Autodesk Inventor part; units mm, degrees
ref_plane "YZ Plane" through (0, 0, 0) normal (1, 0, 0) x (0, 1, 0)
ref_plane "XZ Plane" through (0, 0, 0) normal (0, 1, 0) x (-1, 0, 0)
ref_plane "XY Plane" through (0, 0, 0) normal (0, 0, 1) x (1, 0, 0)
sketch "Sketch1" plane through (0, 0, 0) normal (0, 0, 1) x (1, 0, 0)
  line L0 (-160.1126, 202.6875) -> (-23.9126, 202.6875)
  line L1 (-23.9126, 202.6875) -> (-23.9126, 142.6875)
  line L2 (-23.9126, 142.6875) -> (-163.9126, 142.6875)
  line L3 (-163.9126, 142.6875) -> (-163.9126, 198.8875)
  circle A0 centre (-160.1126, 198.8875) radius 1.5
  arc A1 (-160.1126, 202.6875) -> (-163.9126, 198.8875) centre (-160.1126, 198.8875) ccw
  line L4 (-163.9126, 172.6875) -> (-23.9126, 172.6875) construction
  line L5 (-93.9126, 142.6875) -> (-93.9126, 202.6875) construction
  circle A2 centre (-160.1126, 146.4875) radius 1.5
  circle A3 centre (-27.7126, 198.8875) radius 1.5
  circle A4 centre (-27.7126, 146.4875) radius 1.5
  arc A5 (-163.9126, 146.4875) -> (-160.1126, 142.6875) centre (-160.1126, 146.4875) ccw
  arc A6 (-23.9126, 198.8875) -> (-27.7126, 202.6875) centre (-27.7126, 198.8875) ccw
  arc A7 (-27.7126, 142.6875) -> (-23.9126, 146.4875) centre (-27.7126, 146.4875) ccw
  point P0 (0, 0)
  point P1 (-163.9126, 202.6875)
  dimension "d0" = 60
  dimension "d1" = 140
  dimension "d2" = 3
  dimension "d3" = 3.8
  dimension "d4" = 3.8
  dimension "d5" = 3.8
extrude "Extrusion1" add sketch "Sketch1" along normal blind 1.6 contours L0 A6 L1 A7 L2 A5 L3 A1
sketch "Sketch2" plane through (0, 0, 0) normal (0, 0, -1) x (-1, 0, 0)
  line L0 (139.9626, 193.3375) -> (107.8626, 193.3375)
  line L1 (107.8626, 193.3375) -> (107.8626, 152.0375) construction
  line L2 (107.8626, 152.0375) -> (139.9626, 152.0375)
  line L3 (139.9626, 152.0375) -> (139.9626, 193.3375)
  line L4 (139.9626, 172.6875) -> (107.8626, 172.6875) construction
  line L5 (117.8626, 176.1875) -> (107.8626, 176.1875)
  line L6 (107.8626, 176.1875) -> (107.8626, 169.1875) construction
  line L7 (107.8626, 169.1875) -> (117.8626, 169.1875)
  line L8 (117.8626, 169.1875) -> (117.8626, 176.1875) construction
  line L9 (117.8626, 176.1875) -> (107.8626, 169.1875) construction
  line L10 (107.8626, 176.1875) -> (117.8626, 169.1875) construction
  line L11 (107.8626, 193.3375) -> (107.8626, 176.1875)
  line L12 (107.8626, 169.1875) -> (107.8626, 152.0375)
  line L13 (93.9126, 174.1875) -> (117.8626, 174.1875)
  line L14 (117.8626, 174.1875) -> (117.8626, 171.1875) construction
  line L15 (117.8626, 171.1875) -> (93.9126, 171.1875)
  line L16 (93.9126, 171.1875) -> (93.9126, 174.1875)
  line L17 (93.9126, 174.1875) -> (117.8626, 171.1875) construction
  line L18 (117.8626, 174.1875) -> (93.9126, 171.1875) construction
  line L19 (117.8626, 174.1875) -> (117.8626, 176.1875)
  line L20 (27.7126, 202.6875) -> (160.1126, 202.6875)
  line L21 (160.1126, 142.6875) -> (27.7126, 142.6875)
  line L22 (27.7126, 202.6875) -> (160.1126, 202.6875)
  line L23 (93.9126, 202.6875) -> (93.9126, 142.6875) construction
  line L24 (163.9126, 198.8875) -> (163.9126, 146.4875)
  line L25 (163.9126, 172.6875) -> (23.9126, 172.6875) construction
  line L26 (23.9126, 146.4875) -> (23.9126, 198.8875)
  line L27 (123.9126, 193.3375) -> (123.9126, 152.0375) construction
  line L28 (47.8626, 193.3375) -> (79.9626, 193.3375)
  line L29 (79.9626, 193.3375) -> (79.9626, 152.0375) construction
  line L30 (79.9626, 152.0375) -> (47.8626, 152.0375)
  line L31 (47.8626, 152.0375) -> (47.8626, 193.3375)
  line L32 (47.8626, 172.6875) -> (79.9626, 172.6875) construction
  line L33 (69.9626, 176.1875) -> (79.9626, 176.1875)
  line L34 (79.9626, 176.1875) -> (79.9626, 169.1875) construction
  line L35 (79.9626, 169.1875) -> (69.9626, 169.1875)
  line L36 (69.9626, 169.1875) -> (69.9626, 176.1875) construction
  line L37 (69.9626, 176.1875) -> (79.9626, 169.1875) construction
  line L38 (79.9626, 176.1875) -> (69.9626, 169.1875) construction
  line L39 (79.9626, 193.3375) -> (79.9626, 176.1875)
  line L40 (79.9626, 169.1875) -> (79.9626, 152.0375)
  line L41 (93.9126, 174.1875) -> (69.9626, 174.1875)
  line L42 (69.9626, 174.1875) -> (69.9626, 171.1875) construction
  line L43 (69.9626, 171.1875) -> (93.9126, 171.1875)
  line L44 (69.9626, 174.1875) -> (69.9626, 176.1875)
  line L45 (63.9126, 193.3375) -> (63.9126, 152.0375) construction
  line L46 (117.8626, 171.1875) -> (117.8626, 169.1875)
  line L47 (69.9626, 171.1875) -> (69.9626, 169.1875)
  point P0 (0, 0)
  point P1 (112.8626, 172.6875)
  point P2 (105.8876, 172.6875)
  point P3 (93.9126, 172.6875)
  point P4 (74.9626, 172.6875)
  point P5 (81.9376, 172.6875)
  dimension "d8" = 41.3
  dimension "d9" = 32.1
  dimension "d10" = 10
  dimension "d11" = 3
  dimension "d12" = 7
  dimension "d13" = 30
extrude "Extrusion2" add sketch "Sketch2" along normal blind 0.035
properties part number "Phased_array"
Here's how the part is built. I have some questions about the finished solid (model axes, mm). Give positions to 0.01 mm unless a question says otherwise; leave off trailing zeros. Use one line per item in the form item = value. Start each with the question number.
Q1. I need wall thicknesses on line 1 along X through (y, z) = (199, 0.35); line 2 along Z through (x, y) = (-38, 152.5); line 3 along X through (y, z) = (198, 0.7). Which ranges of each line are inside material? Lowest first, please.
Q2. Thinking about a two-plate mould opening in X: for faces 1 (the cylindrical face through (-28.04, 200.35, 0.79)), 2 (the flat face through (-95, 173, 1.6)), 3 (the cylindrical face through (-162.8, 143.8, 0.8)), which applies, +X half, -X half, draft (parallel to the pull), parting line (faces both ways), or undercut?
Q3. Will this pin go through, and if not, where does the flat tip stop? pin 1 Ø4 at (x, y) = (-160.11, 198.89) entering from -Z.
Taken from the geometry:
q1.line_1 = -163.91 to -161.61, -158.62 to -29.21, -26.22 to -23.91
q1.line_2 = 0 to 1.6
q1.line_3 = -163.91 to -161.32, -158.9 to -28.92, -26.5 to -23.91
q2.face_1 = undercut
q2.face_2 = draft
q2.face_3 = -X half
q3.pin_1 = 0
